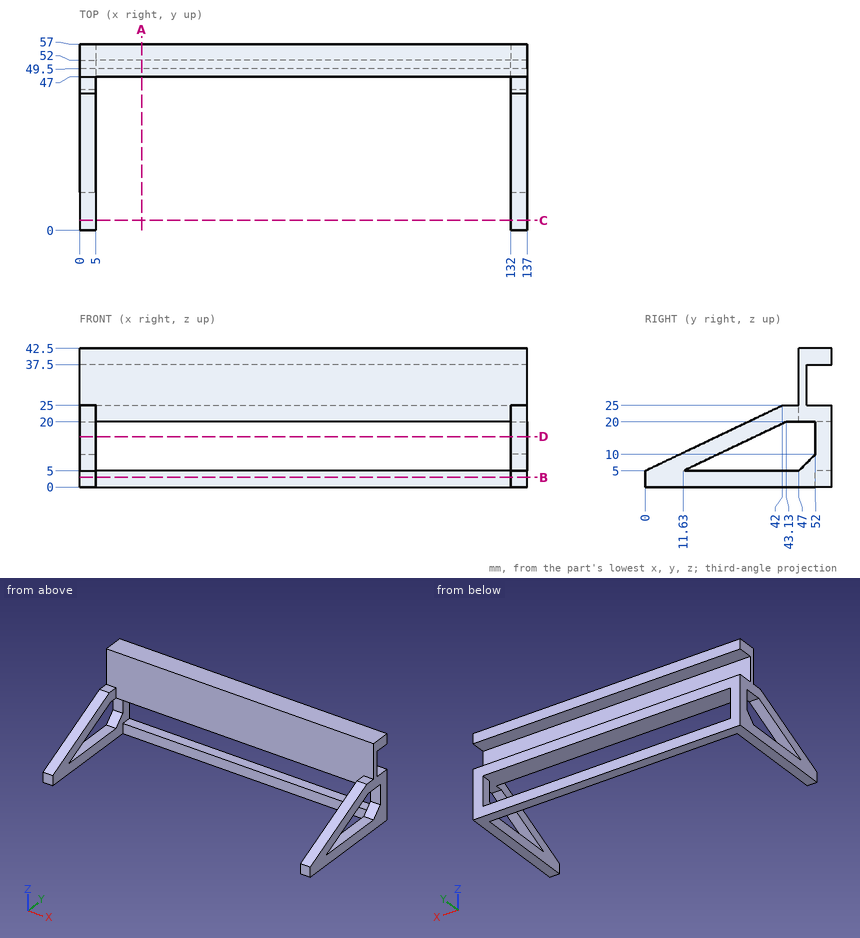
Answer from the drawing. Dimensions are ordinates in mm from the lowest x, y and z of the part. Coordinates: 2 decimals unless noted, no trailing zeros. Write each loop counter-clockwise with the first axis right and the second up, starting at its lowest first coordinate (ties: lowest second). Pieces come first, ordered by that corner, then holes. Notation, with made-up numbers: (-1, 20) - (56, 20) arc R7 cw to (56, 33) - close; hole circle Ø1 at (62, 83). An arc over 180 degrees is marked (long way). Return JSON: item names as keys, results as strings.
1. Each of these flat-tipped pins is pushed along its axis until it touches: pin 1 Ø1.5 at (x, y) = (2.5, 44) entering from +Z; pin 2 Ø1.5 at (x, z) = (134, 15) entering from -Y (1 decimal); pin 3 Ø8 at (x, z) = (115, 13) entering from -Y; pin 4 Ø8 at (x, z) = (49.5, 30) entering from +Y. Where does it stop, or does it pass through?
Final values:
{"pin 1": "z = 25", "pin 2": "y = 19.4", "pin 3": "through", "pin 4": "y = 49.5"}
2. The part is cut by section D-D on z = 15.5. Determine the outline of the cut face in (x, y).
Final values:
{"outline": "(0, 22.05) - (5, 22.05) - (5, 33.68) - (0, 33.68) - close; (0, 52) - (5, 52) - (5, 57) - (0, 57) - close; (132, 22.05) - (137, 22.05) - (137, 33.68) - (132, 33.68) - close; (132, 52) - (137, 52) - (137, 57) - (132, 57) - close"}
3. Consider line 1 along X through (y, z) = (48, 5); line 2 along Y through (x, z) = (22, 23); line 3 along Y through (x, z) = (50.5, 27). Determine where each line is inside the solid, lowest interval first.
Final values:
{"line 1": "0 to 5, 132 to 137", "line 2": "47 to 57", "line 3": "47 to 49.5"}
4. The part is cut by section A-A on x = 19. Determine the outline of the cut face in (y, z), then the cut area to 3 significant figures.
Final values:
{"outline": "(47, 20) - (57, 20) - (57, 25) - (49.5, 25) - (49.5, 37.5) - (57, 37.5) - (57, 42.5) - (47, 42.5) - close; (52, 0) - (57, 0) - (57, 5) - (52, 5) - close", "area": "156 mm^2"}
5. The part is cut by section B-B on z = 3. Determine the outline of the cut face in (x, y).
Final values:
{"outline": "(0, 0) - (5, 0) - (5, 52) - (132, 52) - (132, 0) - (137, 0) - (137, 57) - (0, 57) - close"}
6. The part is cut by section C-C on y = 3. Determine the outline of the cut face in (x, z).
Final values:
{"outline": "(0, 0) - (5, 0) - (5, 6.43) - (0, 6.43) - close; (132, 0) - (137, 0) - (137, 6.43) - (132, 6.43) - close"}
